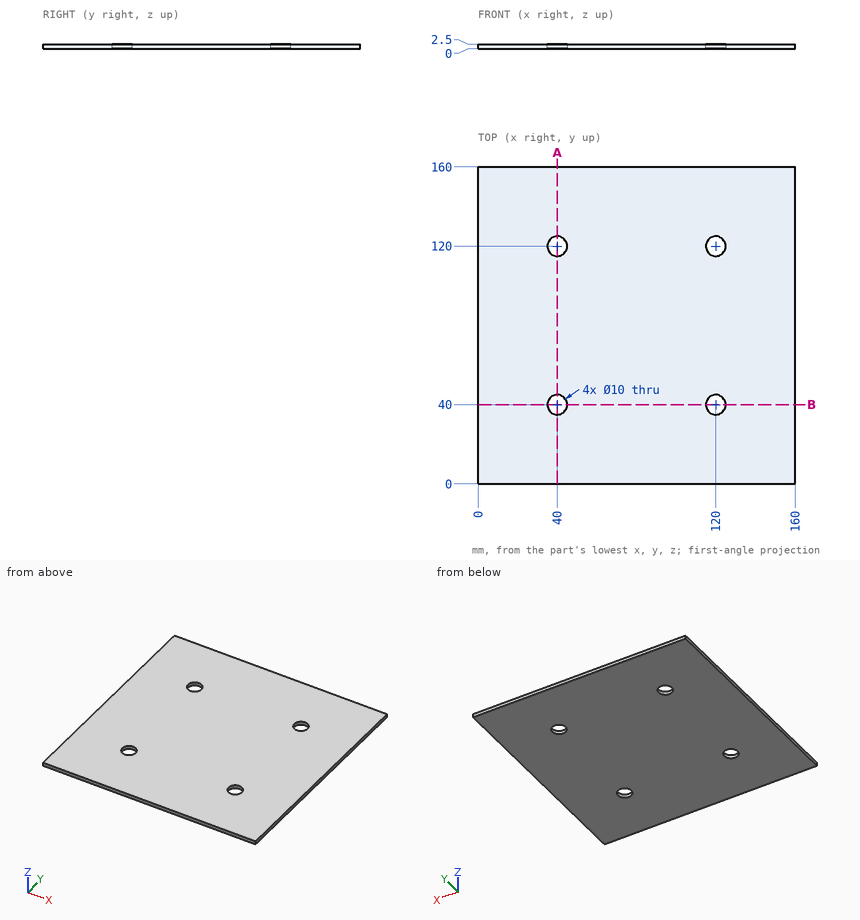
Job drawing, mm, ordinate dimensions from the low corner. One solid piece. Coordinates: 2 decimals unless noted, no trailing zeros. Loops run counter-clockwise (first coordinate to the right, second up) from the corner with the lowest first, then second, coordinate; pieces in that order, holes last. Notation, with made-up numbers: (12, 85) - (62, 85) arc R13 cw to (62, 90) - close; hole circle Ø7 at (32, 31). An arc over 180 degrees is marked (long way). Answer as a JSON object with one key per item and string values. Group by question number.
(1) Cut at A-A (x = 40). Give the cut face in (y, z).
(2) Probe line 1 along Y through (x, z) = (120, 1.85); line 2 along Y through (x, z) = (116, 1.9); line 3 along X through (y, z) = (41, 2). List the from-to ranges inside material, lowest first.
Geometry says:
{
 "1": {"outline": "(0, 0) - (35, 0) - (35, 2.5) - (0, 2.5) - close; (45, 0) - (115, 0) - (115, 2.5) - (45, 2.5) - close; (125, 0) - (160, 0) - (160, 2.5) - (125, 2.5) - close"},
 "2": {"line 1": "y = 0 to 35, 45 to 115, 125 to 160", "line 2": "y = 0 to 37, 43 to 117, 123 to 160", "line 3": "x = 0 to 35.1, 44.9 to 115.1, 124.9 to 160"}
}
